Can you work these out from the model? Positions are in its coordinate system, mm. A direction names the side the tool comes from. Give positions to 0.01 mm unless a question says otherwise; leave off trailing zeros. Order: outer loops, then holes, each group sorted by start corner. A loop starts at its lowest first (then second) coordinate and runs counter-clockwise, first axis right, second up.
Item 1: I want a section at B-B, the plane y = -15.5. Write out the boundary of the cut face in (x, z), then the cut area to 3 significant figures.
Item 2: I want a section at A-A, the plane y = 15. Write out the boundary of the cut face in (x, z).
Item 3: If I drill on line 1 along Z through (x, y) = (2, -17), over which ranges is the centre line in solid material (lowest first)?
Item 4: Which directions (+Z, -Z, +X, -X, +Y, -Y) give clear straight access to the entire face, cutting with the end or side of a thin tool? Please do faces 1 (the cylindrical face through (9.139, -14.334, 36.493)), 2 (the flat face through (0, 0, 37)).
Solid Edge part; units mm, degrees
sketch "Sketch1" plane through (0, 0, 0) normal (0, 0, 1) x (1, 0, 0)
  line L0 (-19, -19) -> (19, -19)
  line L1 (19, -19) -> (19, 19)
  line L2 (19, 19) -> (-19, 19)
  line L3 (-19, 19) -> (-19, -19)
extrude "Protrusion1" add sketch "Sketch1" along normal blind 36
sketch "Sketch2" plane through (0, 0, 36) normal (0, 0, 1) x (1, 0, 0)
  circle A0 centre (0, 0) radius 17
extrude "ExtrudedProtrusion_2" add sketch "Sketch2" along normal blind 1
Results list:
1. outline: (-19, 0) - (19, 0) - (19, 36) - (6.98, 36) - (6.98, 37) - (-6.98, 37) - (-6.98, 36) - (-19, 36) - close
1. area: 1,380 mm2
2. outline: (-19, 0) - (19, 0) - (19, 36) - (8, 36) - (8, 37) - (-8, 37) - (-8, 36) - (-19, 36) - close
3. line 1: z = 0 to 36
4. face 1: +Z
4. face 2: +Z, +X, -X, +Y, -Y
